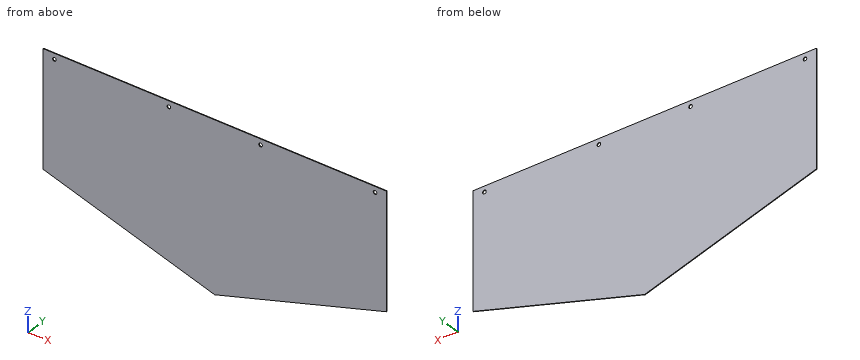
from build123d import *

# Parameters (mm, degrees)
BOSS_EXTRUDE1_DEPTH              = 3.175
F_5_8_0_625_DIAMETER_HOLE1_D     = 15.875
F_5_8_0_625_DIAMETER_HOLE1_DEPTH = 3.175


with BuildPart() as part:
    # Sketch1 → Boss-Extrude1 (new body)
    with BuildSketch(Plane(origin=(0, 0, 0), x_dir=(1, 0, 0), z_dir=(0, 1, 0))):
        Polygon((0, 0), (1524, 0), (1524, 508), (762, 736.6), (0, 508), align=None)
    extrude(amount=BOSS_EXTRUDE1_DEPTH)

    # 5/8 (0.625) Diameter Hole1
    with Locations(Plane.XZ):
        with Locations((50.8, -25.4), (558.8, -25.325960299), (965.2, -25.266728538), (1473.2, -25.192688837)):
            Hole(F_5_8_0_625_DIAMETER_HOLE1_D / 2, depth=F_5_8_0_625_DIAMETER_HOLE1_DEPTH)


solid = part.part
Read the model definition and answer for the solid it produces. Units are mm, in the model's axes. Give positions to 0.01 mm unless a question says otherwise; leave off trailing zeros. Write each loop counter-clockwise with the first axis right and the second up, starting at its lowest first coordinate (ties: lowest second). Pieces come first, ordered by that corner, then holes. Notation, with made-up numbers: (17, 73) - (21, 73) arc R13 ccw to (21, 84) - close; hole circle Ø7 at (85, 54). An arc over 180 degrees is marked (long way). Use CSV: the item, a comma, the result in double quotes. Start each with the question number.
Item 1: The part is cut by section B-B, the plane x = 479.5. Give the vertices of the cut face in (y, z) (3 decimals), and give its area (3 significant figures).
Item 2: The part is cut by section A-A, the plane y = 0.8. Give the vertices of the cut face in (x, z) (1 decimal).
Item 3: Consider line 1 (Z direction, x = 1473.2, y = 2.4); line 2 (Z direction, x = 50.8, y = 2.15); line 3 (Z direction, x = 659.5, y = 1.8). Determine where each line is inside the solid, lowest interval first.
Item 4: Flat-ended cylindrical pins translate along their axes: P1, Ø1, axis at x = 1351.5, y = 2, coming from the -Z side; P2, Ø14.5, axis at x = 50.8, z = -25.4, coming from the -Y side. Find the tip coordinate at first contact, or state that the pin passes through.
Item 5: The part is cut by section C-C, the plane z = -689.5. Give the vertices of the cut face in (x, y) (3 decimals).
Taken from the geometry:
1,outline,"(0, -651.85) - (3.175, -651.85) - (3.175, 0) - (0, 0) - close"
1,area,"2,070 mm2"
2,outline,"(0, -508) - (762, -736.6) - (1524, -508) - (1524, 0) - (0, 0) - close; hole circle Ø15.9 at (50.8, -25.4); hole circle Ø15.9 at (558.8, -25.3); hole circle Ø15.9 at (965.2, -25.3); hole circle Ø15.9 at (1473.2, -25.2)"
3,line 1,"-523.24 to -33.13, -17.26 to 0"
3,line 2,"-523.24 to -33.34, -17.46 to 0"
3,line 3,"-705.85 to 0"
4,P1,"z = -559.9"
4,P2,"through"
5,outline,"(605, 0) - (919, 0) - (919, 3.175) - (605, 3.175) - close"
